CAD build for the part. Positions are in the model's coordinates, mm. A direction names the side the tool comes from. Give positions to 0.01 mm unless a question says otherwise; leave off trailing zeros. Loops run counter-clockwise (first coordinate to the right, second up) from the corner with the lowest first, then second, coordinate; pieces in that order, holes last.
Item 1: Probe probe 1 along Z at (x, y) = (0.5, -1); probe 2 along Y at (x, z) = (0, 4.5); probe 3 along Z at (x, y) = (-1.5, -0.5). List the from-to ranges inside material, lowest first.
Item 2: Which spindle directions (+Z, -Z, +X, -X, +Y, -Y) get a long thin tool onto all of the face, cutting with end or side? Do faces 1 (the flat face through (1.3, -1.3, 6)), 2 (the flat face through (0, 0, 8)). Say none if no direction does.
Item 3: Saw through at A-A on z = -8.5. Give the cut face in (x, y).
Item 4: Drop flat-ended pins along their axis: P1, Ø2, axis at y = 0.5, z = 3.5, coming from the +X side; P2, Ø1, axis at x = -1, y = 1.5, coming from the -Z side. Give the stop position or say it passes through.
Autodesk Inventor part; units mm, degrees
ref_plane "YZ Plane" through (0, 0, 0) normal (1, 0, 0) x (0, 1, 0)
ref_plane "XZ Plane" through (0, 0, 0) normal (0, 1, 0) x (-1, 0, 0)
ref_plane "XY Plane" through (0, 0, 0) normal (0, 0, 1) x (1, 0, 0)
sketch "スケッチ1" plane through (0, 0, 0) normal (0, 0, 1) x (1, 0, 0)
  circle A0 centre (0, 0) radius 1.5
  dimension "d0" = 3
extrude "押し出し1" add sketch "スケッチ1" along normal blind 6
sketch "スケッチ2" plane through (0, 0, 6) normal (0, 0, 1) x (1, 0, 0)
  circle A0 centre (0, 0) radius 1.5
  circle A1 centre (0, 0) radius 3
  dimension "d3" = 6
extrude "押し出し2" add sketch "スケッチ2" along normal blind 2 contours A0 | A1
fillet "フィレット1" radius 2 1 edges at (-3, 0, 8)
thread "ねじ1"
sketch "スケッチ3" plane through (0, 0, 0) normal (0, 0, -1) x (-1, 0, 0)
  circle A0 centre (0, 0) radius 1.5
extrude "押し出し3" add sketch "スケッチ3" along normal blind 9
sketch "スケッチ4" plane through (0, 0, -9) normal (0, 0, -1) x (-1, 0, 0)
  circle A0 centre (0, 0) radius 1.5
extrude "押し出し4" add sketch "スケッチ4" along normal blind 5
properties part number "SB　20mmなべネジ" material "Steel, Mild"
Results below:
1. probe 1: z = -14 to 8
1. probe 2: y = -1.5 to 1.5
1. probe 3: z = 6 to 7.91
2. face 1: -Z
2. face 2: +Z, +X, -X, +Y, -Y
3. outline: circle Ø3 at (0, 0)
4. P1: stops at x = 1.5
4. P2: stops at z = -14
